Geometry: final body of the model. Coordinates: model frame, mm. Face numbers are marked on the shaded views. A direction names the side the tool comes from. Coordinates: 2 decimals unless noted, no trailing zeros. Write each loop counter-clockwise with the first axis right and the second up, starting at its lowest first coordinate (ties: lowest second). Pieces come first, ordered by that corner, then holes. Notation, with made-up numbers: (-4, -31.75) -> (35, -31.75) arc R18 ccw to (35, -27.75) -> close; hole circle Ø8 at (41, 55). An arc over 180 degrees is marked (long way). One line per item, written item: value.
```python
from build123d import *

# Parameters (mm, degrees)
SKETCH_1_R           = 4
EXTRUDE_1_DEPTH      = 52
EXTRUDE_2_DEPTH      = 21
EXTRUDE_2_DEPTH_BACK = 92
SKETCH_2_R           = 3
SKETCH_3_R           = 2.5
EXTRUDE_3_DEPTH      = 5
EXTRUDE_START        = 5
SKETCH_4_R           = 2.5
EXTRUDE_4_DEPTH      = 5


with BuildPart() as part:
    # 草图1 → 凸台-拉伸1 (new body)
    with BuildSketch(Plane.XY):
        with Locations(Location((0, 0, 0), (0, 0, 180))):
            Circle(SKETCH_1_R)
    extrude(amount=EXTRUDE_1_DEPTH)

    # 草图2 → 凸台-拉伸2 (add, two sides: drawn at the far end of the back side and taken through both)
    with BuildSketch(Plane.XY.offset(52).offset(-EXTRUDE_2_DEPTH_BACK)):
        Circle(SKETCH_2_R)
    extrude(amount=EXTRUDE_2_DEPTH + EXTRUDE_2_DEPTH_BACK)

    # 草图3 → 凸台-拉伸3 (add)
    with BuildSketch(Plane(origin=(0, 0, -40), x_dir=(-1, 0, 0), z_dir=(0, 0, -1))):
        Circle(SKETCH_3_R)
    extrude(amount=EXTRUDE_3_DEPTH)

    # 草图4 → 凸台-拉伸4 (add)
    with BuildSketch(Plane.XY.offset(73).offset(EXTRUDE_START)):
        with Locations(Location((0, 0, 0), (0, 0, 180))):
            Circle(SKETCH_4_R)
    extrude(amount=-EXTRUDE_4_DEPTH)


solid = part.part
```
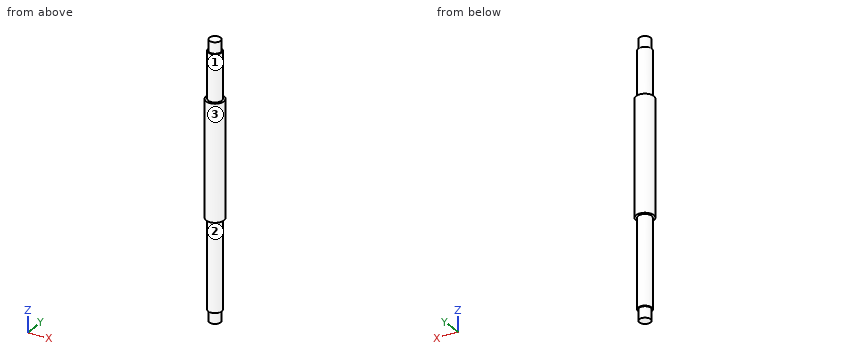
(1) First-contact query: pin 1 (2 mm diameter, centred on x = -3, z = 4.5, fed in from +Y); pin 2 (1 mm diameter, centred on x = -3, y = 2, fed in from -Z). Flat tips, straight axial feed; report the tip coordinate or a pass-through.
Responses:
pin 1: stops at y = 3.46
pin 2: stops at z = 0
(2) Section A-A (x = -0.75). Return the cut outline in (y, z).
Responses:
outline: (-3.93, 0) -> (-2.9, 0) -> (-2.9, -40) -> (-2.38, -40) -> (-2.38, -45) -> (2.38, -45) -> (2.38, -40) -> (2.9, -40) -> (2.9, 0) -> (3.93, 0) -> (3.93, 52) -> (2.9, 52) -> (2.9, 73) -> (2.38, 73) -> (2.38, 78) -> (-2.38, 78) -> (-2.38, 73) -> (-2.9, 73) -> (-2.9, 52) -> (-3.93, 52) -> close
(3) Section C-C (z = 9). Return the cut outline in (x, y), then the cut area to 3 significant figures.
Responses:
outline: circle Ø8 at (0, 0)
area: 50.3 mm2
(4) Section B-B (y = 0). Return the cut outline in (x, z).
Responses:
outline: (-4, 0) -> (-3, 0) -> (-3, -40) -> (-2.5, -40) -> (-2.5, -45) -> (2.5, -45) -> (2.5, -40) -> (3, -40) -> (3, 0) -> (4, 0) -> (4, 52) -> (3, 52) -> (3, 73) -> (2.5, 73) -> (2.5, 78) -> (-2.5, 78) -> (-2.5, 73) -> (-3, 73) -> (-3, 52) -> (-4, 52) -> close
(5) Line query: line 1 (Y direction, x = 0, z = -33); line 2 (Z direction, x = -3, y = -1); line 3 (Z direction, x = 2.25, y = 1.5). Output: solid intervals per line, ascending. Write a range as [from, to].
Responses:
line 1: y = [-3, 3]
line 2: z = [0, 52]
line 3: z = [-40, 73]
(6) Reachability of the marked faces 1, 2 and 3 from +Z, -Z, +X, -X, +Y, -Y: full face, straight path, thin tool, end or side. Return the list, or none.
Responses:
face 1: +Z
face 2: -Z
face 3: +Z, -Z
